```python
from build123d import *

# Parameters (mm, degrees)
SKETCH1_W           = 200
SKETCH1_H           = 100
SKETCH1_R           = 2.5
SKETCH1_W_2         = 120.5
SKETCH1_H_2         = 64
BOSS_EXTRUDE1_DEPTH = 3.175
SKETCH2_R           = 2.5
CUT_EXTRUDE1_DEPTH  = 112.848471715


with BuildPart() as part:
    # Sketch1 → Boss-Extrude1 (new body)
    # profile 1 of 2: a face of its own
    with BuildSketch(Plane(origin=(0, 0, 0), x_dir=(1, 0, 0), z_dir=(0, 1, 0))):
        Rectangle(SKETCH1_W, SKETCH1_H)
        with Locations(Location((90, -40, 0), (0, 0, 270))):
            Circle(SKETCH1_R, mode=Mode.SUBTRACT)
        with Locations(Location((-90, -40, 0), (0, 0, 270))):
            Circle(SKETCH1_R, mode=Mode.SUBTRACT)
        with Locations(Location((-90, 40, 0), (0, 0, 270))):
            Circle(SKETCH1_R, mode=Mode.SUBTRACT)
        with Locations(Location((90, 40, 0), (0, 0, 270))):
            Circle(SKETCH1_R, mode=Mode.SUBTRACT)
        Rectangle(SKETCH1_W_2, SKETCH1_H_2, mode=Mode.SUBTRACT)
    # profile 2 of 2: a face of its own
    with BuildSketch(Plane(origin=(0, 0, 0), x_dir=(1, 0, 0), z_dir=(0, 1, 0))):
        Rectangle(SKETCH1_W_2, SKETCH1_H_2)
    extrude(amount=BOSS_EXTRUDE1_DEPTH)

    # Sketch2 → Cut-Extrude1 (cut, through all)
    with BuildSketch(Plane(origin=(0, 3.175, 0), x_dir=(1, 0, 0), z_dir=(0, 1, 0))):
        with Locations(Location((-78, 0, 0), (0, 0, 270))):
            Circle(SKETCH2_R)
        with Locations(Location((78, 0, 0), (0, 0, 90))):
            Circle(SKETCH2_R)
    extrude(amount=-CUT_EXTRUDE1_DEPTH, mode=Mode.SUBTRACT)


solid = part.part
```
Geometry: final body of the model. Coordinates: model frame, mm. Round coordinates to 2 decimals unless told otherwise and drop trailing zeros. Order: outer loops, then holes, each group sorted by start corner. A loop starts at its lowest first (then second) coordinate and runs counter-clockwise, first axis right, second up. Notation, with made-up numbers: (13.5, -15) -> (44.5, -15) arc R7 cw to (44.5, -11) -> close; hole circle Ø3 at (56, 75). An arc over 180 degrees is marked (long way). Use CSV: the item, a comma, the result in double quotes. Start each with the question number.
1) Section B-B (z = 40). Return the cut outline in (x, y) (3 decimals).
2) Section A-A (x = -90). Return the cut outline in (y, z) (3 decimals).
3) Draft query along X for faces 1 (the face through (-80.22, 1.61, 1.15)), 2 (the face through (-1, 3.175, -1)). Return one class per face: +X half, -X half, draft (parallel to the pull), parting line (faces both ways), or undercut.
4) Material intervals for line 1 along X through (y, z) = (1.1, 0); line 2 along X through (y, z) = (1.6, 40); line 3 along Z through (x, y) = (76, 2.45), sorted ascending. Write a range as from..to.
Returned:
1,outline,"(-100, 0) -> (-92.5, 0) -> (-92.5, 3.175) -> (-100, 3.175) -> close; (-87.5, 0) -> (87.5, 0) -> (87.5, 3.175) -> (-87.5, 3.175) -> close; (92.5, 0) -> (100, 0) -> (100, 3.175) -> (92.5, 3.175) -> close"
2,outline,"(0, -50) -> (3.175, -50) -> (3.175, -42.5) -> (0, -42.5) -> close; (0, -37.5) -> (3.175, -37.5) -> (3.175, 37.5) -> (0, 37.5) -> close; (0, 42.5) -> (3.175, 42.5) -> (3.175, 50) -> (0, 50) -> close"
3,face 1,"undercut"
3,face 2,"draft"
4,line 1,"x = -100..-80.5, -75.5..75.5, 80.5..100"
4,line 2,"x = -100..-92.5, -87.5..87.5, 92.5..100"
4,line 3,"z = -50..-1.5, 1.5..50"
